```python
from build123d import *

# Parameters (mm, degrees)
F0_W     = 12.7
F0_H     = 12.7
F0_W_2   = 50.8
F1_DEPTH = 63.5


with BuildPart() as f1:
    # F0 (on Front) → F1 (new body)
    with BuildSketch(Plane.XZ):
        with Locations((69.85, -57.15)):
            Rectangle(F0_W, F0_H)
        with Locations((38.1, -57.15)):
            Rectangle(F0_W_2, F0_H)
        Polygon((12.7, 0), (0, 0), (0, -63.5), (12.7, -63.5), (12.7, -50.8), align=None)
    extrude(amount=-F1_DEPTH)


solid = f1.part
```
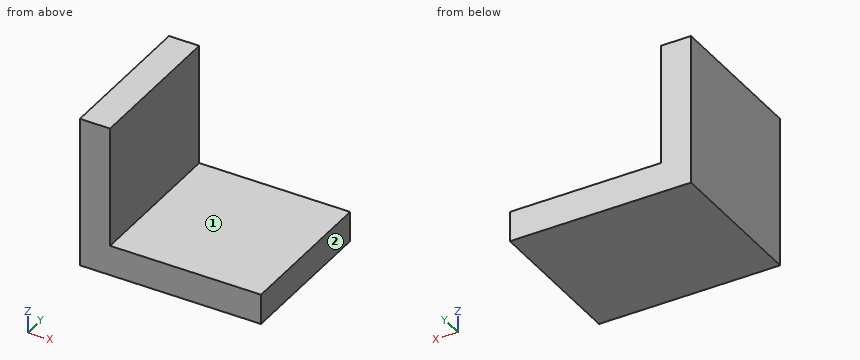
Source: CAD feature listing. Evaluate the final solid. Frame: model axes, mm. Face numbers are marked on the shaded views. A direction names the side the tool comes from. Give positions to 0.01 mm unless a question says otherwise; leave off trailing zeros. Write each loop counter-clockwise with the first axis right and the second up, starting at its lowest first coordinate (ties: lowest second). Pieces come first, ordered by that corner, then holes.
1. Material intervals for line 1 along Z through (x, y) = (57.5, 11); line 2 along X through (y, z) = (51.5, -41.5), sorted ascending.
2. Section query C-C (z = -30.5). Return the cut outline in (x, y).
3. First-contact query: pin 1 (1 mm diameter, centred on y = 17, z = -26, fed in from +X); pin 2 (10 mm diameter, centred on y = 14.5, z = -47, fed in from -X); pin 3 (19 mm diameter, centred on x = 35.5, y = 21.5, fed in from +Z). Flat tips, straight axial feed; report the tip coordinate or a pass-through.
4. Access query for the marked faces 1 and 2. Directions: +Z, -Z, +X, -X, +Y, -Y. A direction counts if a zero-diameter tool reaches every point of the face in a straight line with its end or side. Return the directions, or none.
5. Section query A-A (y = 27). Return the cut outline in (x, z), then the cut area to 3 significant figures.
6. Section query B-B (x = 35.5). Return the cut outline in (y, z).
Output values:
1. line 1: z = -63.5 to -50.8
1. line 2: x = 0 to 12.7
2. outline: (0, 0) - (12.7, 0) - (12.7, 63.5) - (0, 63.5) - close
3. pin 1: stops at x = 12.7
3. pin 2: stops at x = 0
3. pin 3: stops at z = -50.8
4. face 1: +Z, +X, +Y, -Y
4. face 2: +Z, -Z, +X, +Y, -Y
5. outline: (0, -63.5) - (76.2, -63.5) - (76.2, -50.8) - (12.7, -50.8) - (12.7, 0) - (0, 0) - close
5. area: 1,610 mm2
6. outline: (0, -63.5) - (63.5, -63.5) - (63.5, -50.8) - (0, -50.8) - close
